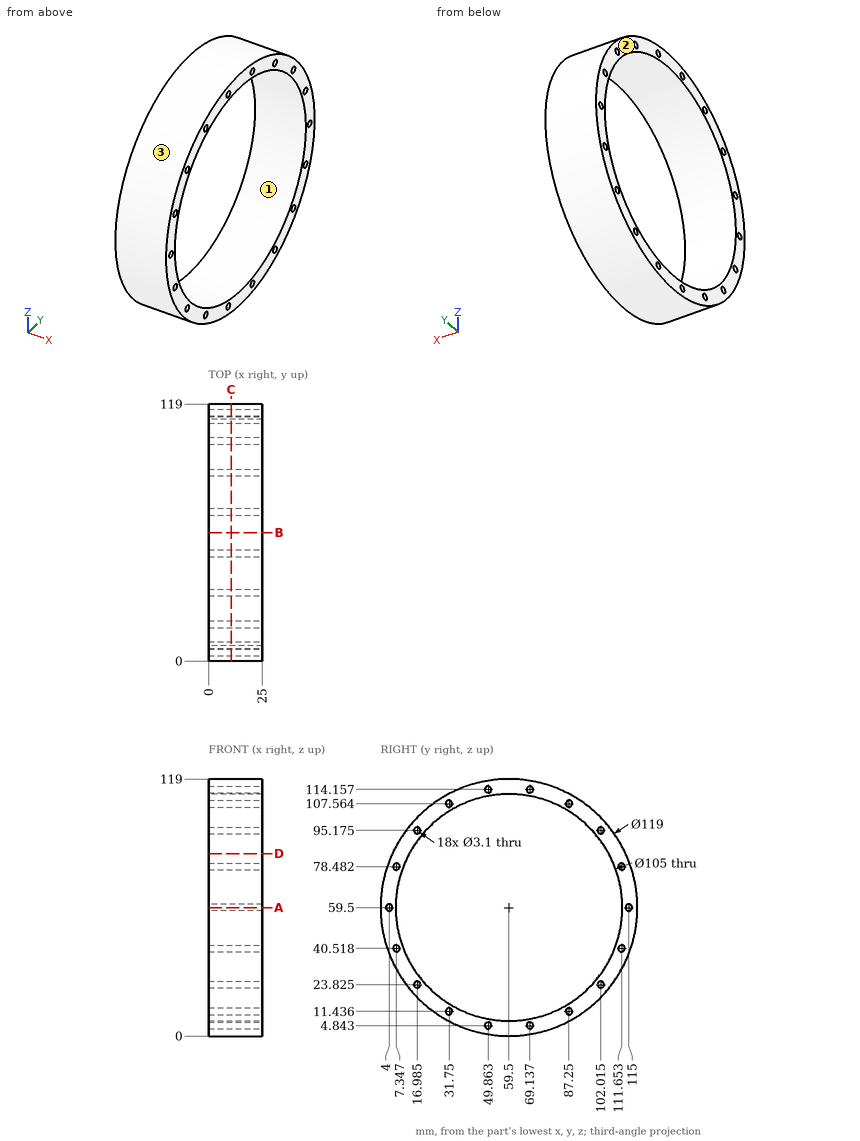
Answer from the drawing. Dimensions are ordinates in mm from the lowest x, y and z of the part. Coordinates: 2 decimals unless noted, no trailing zeros. Write each loop counter-clockwise with the first axis right and the second up, starting at its lowest first coordinate (ties: lowest second). Pieces come first, ordered by that corner, then holes. Notation, with made-up numbers: (-10.5, 89) -> (11.5, 89) arc R20 ccw to (11.5, 98) -> close; hole circle Ø4 at (34.25, 3). An arc over 180 degrees is marked (long way). One line per question, with ' | ' between items.
1. Given pin 1 Ø1 at (x, z) = (3.5, 100.5) entering from +Y; pin 2 Ø3.5 at (y, z) = (87.25, 11.44) entering from +X; pin 3 Ø12 at (x, y) = (14.5, 73) entering from -Z (1 decimal); pin 4 Ø1 at (x, z) = (5, 66.5) entering from -Y, each flat-ended and moving along its own axis, determine where each tip first touches the part or whether it passes through.
Verdict:
pin 1: stops at y = 103.09 | pin 2: stops at x = 25 | pin 3: stops at z = 0.5 | pin 4: stops at y = 0.36
2. For a pull along Y with two mould halves and no side action, classify the marked faces 1, 2 and 3 as released by +Y, released by -Y, zero draft, split by the parting line, or undercut.
Verdict:
face 1: undercut | face 2: zero draft | face 3: split by the parting line
3. Section A-A (z = 59.5) is taken. Determine the outline of the cut face in (x, y).
Verdict:
outline: (0, 0) -> (25, 0) -> (25, 2.45) -> (0, 2.45) -> close; (0, 5.55) -> (25, 5.55) -> (25, 7) -> (0, 7) -> close; (0, 112) -> (25, 112) -> (25, 113.45) -> (0, 113.45) -> close; (0, 116.55) -> (25, 116.55) -> (25, 119) -> (0, 119) -> close
4. Section D-D (z = 84.5) is taken. Determine the outline of the cut face in (x, y) (1 decimal).
Verdict:
outline: (0, 5.5) -> (25, 5.5) -> (25, 13.3) -> (0, 13.3) -> close; (0, 105.7) -> (25, 105.7) -> (25, 113.5) -> (0, 113.5) -> close
5. Straight lines are drawn through the part: line 1 (Z direction, x = 24, y = 49) (1 decimal); line 2 (Z direction, x = 3.75, y = 58); line 3 (Y direction, x = 16, z = 12) (1 decimal). For each, find the intervals that lie inside material, in ascending order.
Verdict:
line 1: z = 0.9 to 3.6, 6.1 to 8.1, 110.9 to 112.9, 115.4 to 118.1 | line 2: z = 0.02 to 7.02, 111.98 to 118.98 | line 3: y = 23.7 to 30.3, 33.2 to 37.1, 81.9 to 85.8, 88.7 to 95.3
6. Section B-B (y = 59.5) is taken. Determine the outline of the cut face in (x, z), and give its area (3 significant figures).
Verdict:
outline: (0, 0) -> (25, 0) -> (25, 7) -> (0, 7) -> close; (0, 112) -> (25, 112) -> (25, 119) -> (0, 119) -> close | area: 350 mm^2
7. Section C-C (x = 10.5) is taken. State how many separate pieces and enclosed holes the cut face has, and give its area (3 significant figures).
Verdict:
separate pieces: 1 | enclosed holes: 19 | area: 2,330 mm^2
